from build123d import *

# Parameters (mm, degrees)
SKETCH_1_R          = 11
EXTRUDE_1_DEPTH     = 2
SKETCH_2_R          = 5
EXTRUDE_2_DEPTH     = 10
SKETCH_3_R          = 3
CUT_EXTRUDE_2_DEPTH = 13
SKETCH_4_R          = 1.5
CUT_EXTRUDE_3_DEPTH = 10
SKETCH_5_R          = 1.5
CUT_EXTRUDE_4_DEPTH = 12


with BuildPart() as part:
    # Эскиз1 → Бобышка-Вытянуть1 (new body)
    with BuildSketch(Plane.XY):
        Circle(SKETCH_1_R)
    extrude(amount=EXTRUDE_1_DEPTH)

    # Эскиз2 → Бобышка-Вытянуть2 (add)
    with BuildSketch(Plane.XY.offset(2)):
        Circle(SKETCH_2_R)
    extrude(amount=EXTRUDE_2_DEPTH)

    # Эскиз3 → Вырез-Вытянуть2 (cut, through all)
    with BuildSketch(Plane.XY):
        Circle(SKETCH_3_R)
    extrude(amount=CUT_EXTRUDE_2_DEPTH, mode=Mode.SUBTRACT)

    # Эскиз4 → Вырез-Вытянуть3 (cut)
    with BuildSketch(Plane.XY.offset(2)):
        with Locations((5.656854249, 5.656854249)):
            Circle(SKETCH_4_R)
        with Locations((5.656854249, -5.656854249)):
            Circle(SKETCH_4_R)
        with Locations((-5.656854249, -5.656854249)):
            Circle(SKETCH_4_R)
        with Locations((-5.656854249, 5.656854249)):
            Circle(SKETCH_4_R)
    extrude(amount=-CUT_EXTRUDE_3_DEPTH, mode=Mode.SUBTRACT)

    # Эскиз5 → Вырез-Вытянуть4 (cut, through all)
    with BuildSketch(Plane(origin=(0, 0, 0), x_dir=(0, 0, -1), z_dir=(1, 0, 0))):
        with Locations((-7.5, 0)):
            Circle(SKETCH_5_R)
    extrude(amount=-CUT_EXTRUDE_4_DEPTH, mode=Mode.SUBTRACT)


solid = part.part
Build history of the part. All positions in model axes, mm. A direction names the side the tool comes from. Coordinates: 2 decimals unless noted, no trailing zeros. Order: outer loops, then holes, each group sorted by start corner. A loop starts at its lowest first (then second) coordinate and runs counter-clockwise, first axis right, second up. Notation, with made-up numbers: (-16, 34.25) - (22, 34.25) arc R26 cw to (22, 64.25) - close; hole circle Ø3 at (43.5, 19). An arc over 180 degrees is marked (long way). Put each result on its own line as item: value.
1. Saw through at B-B (y = 0). Write the cut outline in (x, z), and give its area (3 significant figures).
Answer sheet:
outline: (-11, 0) - (-3, 0) - (-3, 6) - (-5, 6) - (-5, 2) - (-11, 2) - close; (-5, 9) - (-3, 9) - (-3, 12) - (-5, 12) - close; (3, 0) - (11, 0) - (11, 2) - (5, 2) - (5, 12) - (3, 12) - close
area: 66.0 mm^2
2. Tool access for faces 1 (the face through (2.86, 0.9, 5.92)), 2 (the face through (2, -5, 2)): list every direction of +Z, -Z, +X, -X, +Y, -Y with a clear straight run to the whole face (end or side of a thin tool).
Answer sheet:
face 1: +Z, -Z
face 2: +Z
3. Saw through at A-A (x = 0). Write the cut outline in (y, z).
Answer sheet:
outline: (-11, 0) - (-3, 0) - (-3, 12) - (-5, 12) - (-5, 2) - (-11, 2) - close; (3, 0) - (11, 0) - (11, 2) - (5, 2) - (5, 12) - (3, 12) - close
4. Saw through at C-C (x = -6). Write the cut outline in (y, z), and give its area (3 significant figures).
Answer sheet:
outline: (-9.22, 0) - (-7.12, 0) - (-7.12, 2) - (-9.22, 2) - close; (-4.2, 0) - (4.2, 0) - (4.2, 2) - (-4.2, 2) - close; (7.12, 0) - (9.22, 0) - (9.22, 2) - (7.12, 2) - close
area: 25.2 mm^2
5. Saw through at D-D (z = 2.5). Write the cut outline in (x, y), and give its area (3 significant figures).
Answer sheet:
outline: circle Ø10 at (0, 0); hole circle Ø6 at (0, 0)
area: 50.3 mm^2
6. Probe line 1 along X through (y, z) = (0, 5.25); line 2 along Y through (x, z) = (0, 1.5); line 3 along Z through (x, y) = (7.5, 0.5). List the from-to ranges inside material, lowest first. Write a range as [from, to].
Answer sheet:
line 1: x = [-5, -3], [3, 5]
line 2: y = [-11, -3], [3, 11]
line 3: z = [0, 2]
7. Pull direction X, two halves, no side cores. Call faces 3 (the face through (-3.78, -1.33, 6.81)), 4 (the face through (-5.85, -4.17, 1.01)), 5 (the face through (4.77, 1.5, 6.93)): pulls with the +X half, pulls with the -X half, needs draft (parallel to the pull), parting line crosses it, or undercut.
Answer sheet:
face 3: needs draft
face 4: undercut
face 5: parting line crosses it
8. Drop flat-ended pins along their axis: P1, Ø4, axis at x = 5.66, y = 5.66, coming from the +Z side; P2, Ø4, axis at y = 0, z = 7.5, coming from the -X side; P3, Ø6, axis at y = 4.5, z = 10.5, coming from the -X side; P4, Ø5.5, axis at x = 0, y = 0, coming from the +Z side. Give the stop position or say it passes through.
Answer sheet:
P1: stops at z = 2
P2: stops at x = -5
P3: stops at x = -4.77
P4: passes through
